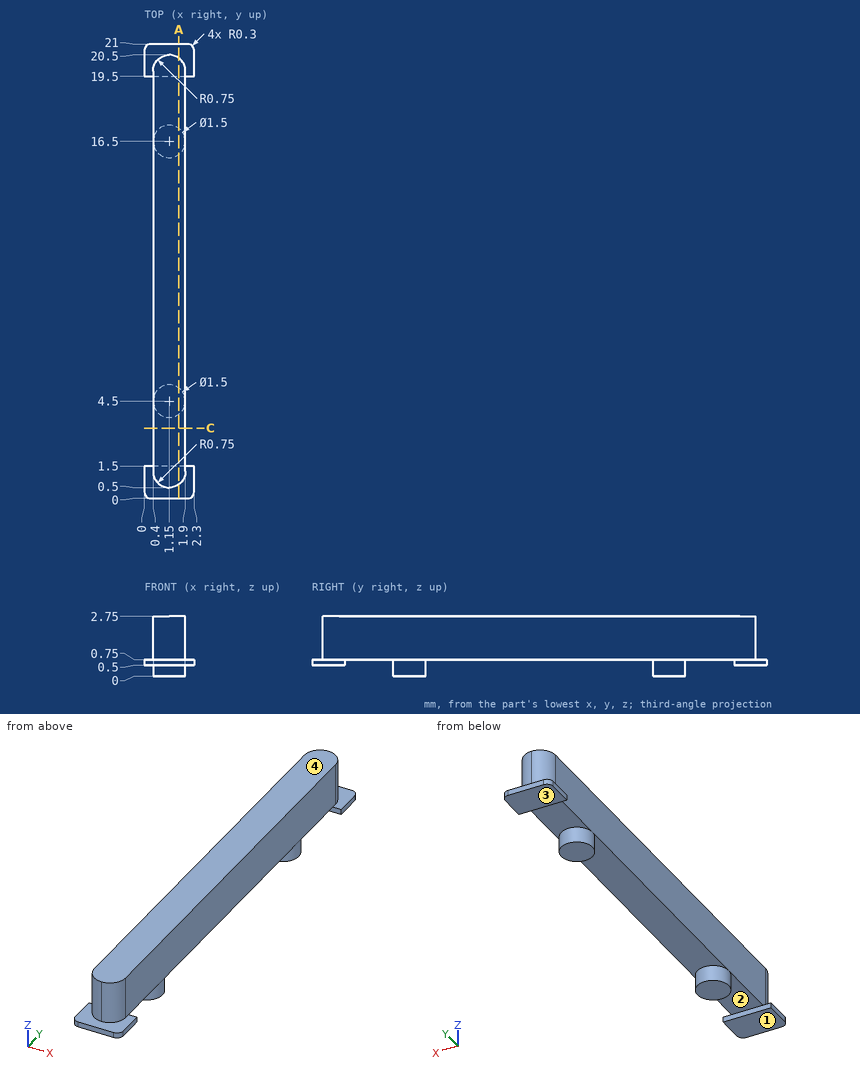
Check sheet for the drawn part. Datum: minimum x, y, z corner. Units: mm. A direction names the side the tool comes from. Give positions to 0.01 mm unless a question says otherwise; leave off trailing zeros. Write each loop counter-clockwise with the first axis right and the second up, starting at its lowest first coordinate (ties: lowest second). Pieces come first, ordered by that corner, then holes. Notation, with made-up numbers: M 72,47 L 118,47 A23 cw 118,86 Z; hole C -4.75,53 d11. An arc over 180 degrees is marked long. One line per question, with ' | ' between items.
1. Cross-section at C-C (y = 3.25). Enter the section's corners in (x, z).
Ans:
outline: M 0.4,0.75 L 1.9,0.75 L 1.9,2.75 L 0.4,2.75 Z
2. Cross-section at A-A (x = 1.6). Enter the section's corners in (y, z), plus the area to 4 significant figures.
Ans:
outline: M 0,0.5 L 1.5,0.5 L 1.5,0.75 L 3.9,0.75 L 3.9,0 L 5.1,0 L 5.1,0.75 L 15.9,0.75 L 15.9,0 L 17.1,0 L 17.1,0.75 L 19.5,0.75 L 19.5,0.5 L 21,0.5 L 21,0.75 L 20.35,0.75 L 20.35,2.75 L 0.65,2.75 L 0.65,0.75 L 0,0.75 Z | area: 41.95 mm2
3. Gauge pin test, flat ends, axial feed: pin 1 (0.8 mm diameter, centred on x = 1, y = 11.5, fed in from -Z); pin 2 (1.2 mm diameter, centred on x = 1.5, y = 1, fed in from -Z); pin 3 (1 mm diameter, centred on y = 8.5, z = 1.5, fed in from +X). Record the tip position at first contact, or that the pin passes through.
Ans:
pin 1: z = 0.75 | pin 2: z = 0.5 | pin 3: x = 1.9
4. Set-up check for the marked faces 3 and 4: record each of +Z, -Z, +X, -X, +Y, -Y from which the full face is reachable in a straight line by a thin tool's end or side.
Ans:
face 3: -Z, +X, -X, +Y | face 4: +Z, +X, -X, +Y, -Y
5. Mould release check, pull along Y, two halves, no side actions. Record for the marked faces 1 and 2: released by +Y, released by -Y, zero draft, split by the parting line, or undercut.
Ans:
face 1: zero draft | face 2: undercut
6. Scan lines: line 1 along Y through (x, z) = (1.4, 0.65); line 2 along X through (y, z) = (3, 2.5); line 3 along Z through (x, y) = (1.8, 17). Record each from-to range of solid material in increasing order. Write a range as from..to.
Ans:
line 1: 0..1.5, 3.79..5.21, 15.79..17.21, 19.5..21 | line 2: 0.4..1.9 | line 3: 0.75..2.75
